Part model, mm, in its own coordinate system. A direction names the side the tool comes from. Round coordinates to 2 decimals unless told otherwise and drop trailing zeros. Write each loop counter-clockwise with the first axis right and the second up, starting at its lowest first coordinate (ties: lowest second). Pieces come first, ordered by that corner, then holes. Notation, with made-up numbers: M -29,82.5 L 8,82.5 A22 cw 8,97.5 Z; hole C -29.5,81 d11. An arc over 180 degrees is marked long. Use a Markdown table: item, result. Add a question column.
1) Slice it at A-A on y = 12.5. Write the cut outline in (x, z), plus the area to 3 significant figures.
2) Which spindle directions (+Z, -Z, +X, -X, +Y, -Y) get a long thin tool onto all of the face, cutting with end or side? Do faces 1 (the face through (-0.158, -11.726, 12.544)), 2 (the face through (-0.16, 11.91, 12.63)), 3 (the face through (2.04, -14.41, 29.84)). Say none if no direction does.
3) Wall check: probe 1 along Y at (x, z) = (7, 23); probe 2 along Z at (x, y) = (-8, -7.25); probe 3 along X at (y, z) = (-0.25, 7). Give the ranges that are in metal, low to high.
4) Drop flat-ended pins along their axis: P1, Ø12, axis at x = -8, z = 5, coming from the -Y side; P2, Ø4, axis at y = -10, z = 9, coming from the +X side; P3, Ø3, axis at y = 9, z = 8.5, coming from the +X side. Give the stop position or say it passes through.
5) Two-plate mould, pull along X, no slides. Class faces 4 (the face through (-11.24, -0.49, 6.59)), 5 (the face through (0, 0, 0)), 6 (the face through (-11.25, 0, 25)), 7 (the face through (10.55, 0.19, 19.93)): released by +X, released by -X, zero draft, split by the parting line, or undercut.
Autodesk Inventor part; units mm, degrees
ref_plane "YZ Plane" through (0, 0, 0) normal (1, 0, 0) x (0, 1, 0)
ref_plane "XZ Plane" through (0, 0, 0) normal (0, 1, 0) x (-1, 0, 0)
ref_plane "XY Plane" through (0, 0, 0) normal (0, 0, 1) x (1, 0, 0)
sketch "Sketch1" plane through (0, 0, 0) normal (1, 0, 0) x (0, 1, 0)
  circle A0 centre (0, 38.3) radius 28.3
  line L0 (-15, 14.3023) -> (15, 14.3023)
  line L1 (15, 14.3023) -> (15, 39.3023)
  line L2 (15, 39.3023) -> (-15, 39.3023)
  line L3 (-15, 39.3023) -> (-15, 14.3023)
  point P0 (0, 0)
  point P1 (0, 10)
  dimension "d0" = 56.6
  dimension "d1" = 10
  dimension "d2" = 25
  dimension "d3" = 30
extrude "Extrusion1" add sketch "Sketch1" along normal mid plane 22.5 contours L0 A0 | L3 L2 L1 L0
sketch "Sketch2" plane through (0, 0, 0) normal (0, 0, 1) x (1, 0, 0)
  circle A0 centre (0, 0) radius 11.25
  dimension "d6" = 22.5
extrude "Extrusion2" add sketch "Sketch2" along normal up to surface
sketch "Sketch3" plane through (-11.25, 0, 14.3023) normal (0, -1, 0) x (1, 0, 0)
  line L0 (0, 25) -> (22.5, 25)
  line L1 (22.5, 25) -> (22.5, 0)
  line L2 (1, 25) -> (22.5, 3.5)
  line L3 (22.5, 6.3284) -> (21.0858, 4.9142)
  line L4 (0, 0) -> (0, 25)
  point P0 (11.25, -14.3023)
  dimension "d12" = 45
  dimension "d13" = 1
  dimension "d14" = 2
extrude "Extrusion3" cut sketch "Sketch3" along normal mid plane 27.6 contours L0 L1 L3 L2
sketch "Sketch4" plane through (0, 0, 0) normal (0, 1, 0) x (-1, 0, 0)
  line L0 (-11.25, 14.3023) -> (-11.25, 39.3023)
  line L1 (-11.25, 20.6307) -> (7.4216, 39.3023)
  line L2 (10.25, 39.3023) -> (-11.25, 39.3023)
  line L3 (-9.8358, 19.2165) -> (10.25, 39.3023)
  point P0 (0, 0)
extrude "Extrusion4" cut sketch "Sketch4" along normal through all both and the other way through all
fillet "Fillet1" radius 0.5 2 edges at (-0.2071, 13.8, 29.2594) (-0.2071, -13.8, 29.2594)
chamfer "Chamfer1" distance 1 angle 45 1 edges at (-11.25, 0, 0)
chamfer "Chamfer2" distance 0.5 angle 45 2 edges at (-11.25, 15, 26.8023) (-11.25, -15, 26.8023)
fillet "Fillet2" radius 2 2 edges at (0.25, -15, 14.3023) (0.25, 15, 14.3023)
equation "\"d3\" = width"
equation "\"d10\" = sample_cut"
equation "\"width\" = 30"
properties part number "pld-target-holder" material "ABS Plastic"
Entries:
| question | item | result |
|---|---|---|
| 1 | outline | M -11.25,12.91 L 11.25,12.91 L 11.25,20.63 L 9.84,19.22 L -10.25,39.3 L -11.25,39.3 Z |
| 1 | area | 365 mm^2 |
| 2 | face 1 | -Z, -Y |
| 2 | face 2 | -Z, +Y |
| 2 | face 3 | +Z, +X, +Y, -Y |
| 3 | probe 1 | y = -15 to -13.8, 13.8 to 15 |
| 3 | probe 2 | z = 0.55 to 37.05 |
| 3 | probe 3 | x = -11.25 to 11.25 |
| 4 | P1 | stops at y = -11.07 |
| 4 | P2 | stops at x = 7.91 |
| 4 | P3 | stops at x = 8.39 |
| 5 | face 4 | split by the parting line |
| 5 | face 5 | zero draft |
| 5 | face 6 | released by -X |
| 5 | face 7 | undercut |
